from build123d import *

# Parameters (mm, degrees)
SKETCH1_R           = 1.5
SKETCH1_R_2         = 4
BOSS_EXTRUDE3_DEPTH = 7


with BuildPart() as part:
    # Sketch1 → Boss-Extrude3 (new body)
    with BuildSketch(Plane(origin=(0, 0, 0), x_dir=(0, 0, -1), z_dir=(1, 0, 0))):
        with BuildLine():
            Line((-16.265163927, 11.0728645), (-7.889471404, 2.697171977))
            ThreePointArc((-7.889471404, 2.697171977), (-5.072000749, -2.885001281), (-6.120829891, -9.049314431))
            Line((-6.120829891, -9.049314431), (-9.01992916, -14.530576551))
            ThreePointArc((-9.01992916, -14.530576551), (-9.320687391, -15.40241611), (-9.342398614, -16.32441847))
            Line((-9.342398614, -16.32441847), (-9.027333312, -18.719831292))
            ThreePointArc((-9.027333312, -18.719831292), (-8.031125849, -20.584013921), (-6.052951061, -21.328614951))
            Line((-6.052951061, -21.328614951), (6.052951061, -21.328614951))
            ThreePointArc((6.052951061, -21.328614951), (8.031125849, -20.584013921), (9.027333312, -18.719831292))
            Line((9.027333312, -18.719831292), (9.342398614, -16.32441847))
            ThreePointArc((9.342398614, -16.32441847), (9.320687391, -15.40241611), (9.01992916, -14.530576551))
            Line((9.01992916, -14.530576551), (6.120829891, -9.049314431))
            ThreePointArc((6.120829891, -9.049314431), (5.072000749, -2.885001281), (7.889471404, 2.697171977))
            Line((7.889471404, 2.697171977), (16.265163927, 11.0728645))
            Line((16.265163927, 11.0728645), (16.265163927, 12.376090748))
            ThreePointArc((16.265163927, 12.376090748), (15.386484271, 14.497411092), (13.265163927, 15.376090748))
            Line((13.265163927, 15.376090748), (9.467130834, 15.376090748))
            Line((9.467130834, 15.376090748), (7.071067812, 12.980027727))
            ThreePointArc((7.071067812, 12.980027727), (0, 10.051095538), (-7.071067812, 12.980027727))
            Line((-7.071067812, 12.980027727), (-9.467130834, 15.376090748))
            Line((-9.467130834, 15.376090748), (-13.265163927, 15.376090748))
            ThreePointArc((-13.265163927, 15.376090748), (-15.386484271, 14.497411092), (-16.265163927, 12.376090748))
            Line((-16.265163927, 12.376090748), (-16.265163927, 11.0728645))
        make_face()
        with Locations((-13.189368773, 12.756003002)):
            Circle(SKETCH1_R, mode=Mode.SUBTRACT)
        with Locations((13.189368773, 12.756003002)):
            Circle(SKETCH1_R, mode=Mode.SUBTRACT)
        with Locations((0, -15.376090748)):
            Circle(SKETCH1_R_2, mode=Mode.SUBTRACT)
    extrude(amount=BOSS_EXTRUDE3_DEPTH)


solid = part.part
Check sheet for the modelled part. Datum: model origin and axes. Units: mm. A direction names the side the tool comes from. Give positions to 0.01 mm unless a question says otherwise; leave off trailing zeros. Write each loop counter-clockwise with the first axis right and the second up, starting at its lowest first coordinate (ties: lowest second). Pieces come first, ordered by that corner, then holes. Notation, with made-up numbers: M 67.25,-29 L 84.25,-29 A12 cw 84.25,-11 Z; hole C 22,-33.5 d3. An arc over 180 degrees is marked long. Use one line per item in the form item = value.
(1) Section check A-A on z = 0. Record the boundary of the cut face in (x, y).
Answer block:
outline = M 0,-21.33 L 7,-21.33 L 7,-19.38 L 0,-19.38 Z; M 0,-11.38 L 7,-11.38 L 7,10.05 L 0,10.05 Z
(2) Section check B-B on y = -18. Record the boundary of the cut face in (x, z), plus the area to 3 significant figures.
Answer block:
outline = M 0,-9.12 L 7,-9.12 L 7,-3.02 L 0,-3.02 Z; M 0,3.02 L 7,3.02 L 7,9.12 L 0,9.12 Z
area = 85.4 mm2
(3) Section check D-D on y = -0.5. Record the boundary of the cut face in (x, z), plus the area to 3 significant figures.
Answer block:
outline = M 0,-5.74 L 7,-5.74 L 7,5.74 L 0,5.74 Z
area = 80.4 mm2
(4) Draft check along Y on faces 1 (the cylindrical face through (3.451, 14.474, -15.41)), 2 (the cylindrical face through (3.45, -11.41, 0.52)), 3 (the flat face through (3.451, -17.505, 9.187)). Enter one of: pulls with the +Y half, pulls with the -Y half, needs draft (parallel to the pull), parting line crosses it, or undercut.
Answer block:
face_1 = pulls with the +Y half
face_2 = undercut
face_3 = pulls with the -Y half
(5) Section check C-C on x = 5.5. Record the boundary of the cut face in (y, z), plus the area to 3 significant figures.
Answer block:
outline = M -21.33,-6.05 A3 ccw -18.72,-9.03 L -16.32,-9.34 A3 ccw -14.53,-9.02 L -9.05,-6.12 A10 cw 2.7,-7.89 L 11.07,-16.27 L 12.38,-16.27 A3 ccw 15.38,-13.27 L 15.38,-9.47 L 12.98,-7.07 A10 cw 12.98,7.07 L 15.38,9.47 L 15.38,13.27 A3 ccw 12.38,16.27 L 11.07,16.27 L 2.7,7.89 A10 cw -9.05,6.12 L -14.53,9.02 A3 ccw -16.32,9.34 L -18.72,9.03 A3 ccw -21.33,6.05 Z; hole C -15.38,0 d8; hole C 12.76,-13.19 d3; hole C 12.76,13.19 d3
area = 542 mm2
(6) Tool access check on faces 4 (the flat face through (3.451, 6.944, 12.136)), 5 (the flat face through (3.45, 14.16, 8.25)), 6 (the cylindrical face through (3.45, 13.21, -14.62)). Record the directions out of +Z, -Z, +X, -X, +Y, -Y that give a thin tool (end or side, any length) a straight path to the whole face; none if there is none.
Answer block:
face_4 = +Z, +X, -X
face_5 = +X, -X, +Y
face_6 = +X, -X
(7) Material ranges on line 1 along Z through (x, y) = (3.75, 12.5); line 2 along Z through (x, y) = (2.75, -15.5); line 3 along Z through (x, y) = (3.75, 13), recorded low to high.
Answer block:
line_1 = -16.26 to -14.67, -11.71 to -6.56, 6.56 to 11.71, 14.67 to 16.26
line_2 = -9.34 to -4, 4 to 9.34
line_3 = -16.2 to -14.67, -11.71 to -7.09, 7.09 to 11.71, 14.67 to 16.2
(8) Depth check by flat-ended pin: P1, Ø2.5, axis at y = 12.76, z = -13.19, coming from the +X side; P2, Ø4, axis at x = 3.5, y = 2.5, coming from the -Z side; P3, Ø1.5, axis at x = 2, y = -1, coming from the -Z side; P4, Ø2, axis at x = 2, y = -14, coming from the -Z side. Enter the tip coordinate at first touch or a pass-through.
Answer block:
P1 = through
P2 = -9.69
P3 = -5.85
P4 = -9.22
